Part model, mm, in its own coordinate system. A direction names the side the tool comes from. Round coordinates to 2 decimals unless told otherwise and drop trailing zeros. Write each loop counter-clockwise with the first axis right and the second up, starting at its lowest first coordinate (ties: lowest second). Pieces come first, ordered by that corner, then holes.
1) Drill centre lines: L1, parallel to Z at x = 2.5, y = 10; L2, parallel to Y at x = 6, z = 36; L3, parallel to X at y = 12.25, z = 45. Where is each one in solid material? Low to high.
2) Saw through at D-D on z = 27.5. Write the cut outline in (x, y).
3) Saw through at C-C on y = 6.25. Write the cut outline in (x, z).
4) Saw through at A-A on x = -3. Write the cut outline in (y, z), and give its area (3 significant figures).
5) Which spindle directions (+Z, -Z, +X, -X, +Y, -Y) get a long thin tool onto all of the face, cutting with end or side? Do faces 4 (the flat face through (18.066, 10.278, 24.65)), 5 (the flat face through (0, 10, 10)). Say none if no direction does.
6) Flat gauge pins, fed straight in: pin 1 (2 mm diameter, centred on y = 5, z = 18, fed in from +X); pin 2 (6 mm diameter, centred on y = 14, z = 6, fed in from +X); pin 3 (5 mm diameter, centred on x = 1.5, y = 9.5, fed in from -Z). Where does each tip first touch, or does it go through?
7) Saw through at B-B on z = 7.5. Write the cut outline in (x, y), and give its area (3 significant figures).
8) Pull direction Y, two halves, no side cores. Call faces 1 (the flat face through (-17.934, 10.507, 24.65)), 2 (the flat face through (-6, 8, 0)), 3 (the cylindrical face through (1.08, 5.05, 4.93)): +Y half, -Y half, draft (parallel to the pull), parting line (faces both ways), or undercut.
```python
from build123d import *

# Parameters (mm, degrees)
SALIENTE_EXTRUIR1_DEPTH = 50
CROQUIS3_R              = 5
CORTAR_EXTRUIR1_DEPTH   = 10


with BuildPart() as part:
    # Croquis2 → Saliente-Extruir1 (new body)
    with BuildSketch(Plane.XY):
        Polygon((-24, -0.041121621), (24, 0.041121621), (11.964387631, 20.805170501), (-12.035612369, 20.76404888), align=None)
    extrude(amount=SALIENTE_EXTRUIR1_DEPTH)

    # Croquis3 → Cortar-Extruir1 (cut)
    with BuildSketch(Plane(origin=(0, 0, 0), x_dir=(-1, 0, 0), z_dir=(0, 0, -1))):
        with Locations((0, 9.933048714)):
            Circle(CROQUIS3_R)
    extrude(amount=-CORTAR_EXTRUIR1_DEPTH, mode=Mode.SUBTRACT)


solid = part.part
```
Completed:
1. L1: z = 10 to 50
1. L2: y = 0.01 to 20.79
1. L3: x = -16.93 to 16.92
2. outline: (-24, -0.04) - (24, 0.04) - (11.96, 20.81) - (-12.04, 20.76) - close
3. outline: (-20.38, 0) - (-3.38, 0) - (-3.38, 10) - (3.38, 10) - (3.38, 0) - (20.4, 0) - (20.4, 50) - (-20.38, 50) - close
4. outline: (-0.01, 0) - (5.93, 0) - (5.93, 10) - (13.93, 10) - (13.93, 0) - (20.78, 0) - (20.78, 50) - (-0.01, 50) - close
4. area: 959 mm2
5. face 4: +Z, -Z, +X, +Y
5. face 5: -Z
6. pin 1: stops at x = 21.71
6. pin 2: stops at x = 17.65
6. pin 3: stops at z = 10
7. outline: (-24, -0.04) - (24, 0.04) - (11.96, 20.81) - (-12.04, 20.76) - close; hole circle Ø10 at (0, 9.93)
7. area: 670 mm2
8. face 1: +Y half
8. face 2: draft
8. face 3: undercut
